```python
from build123d import *

# Parameters (mm, degrees)
SZKIC1_W                    = 32
SZKIC1_H                    = 25
DODANIE_WYCI_GNI_CIE1_DEPTH = 2
SZKIC2_W                    = 5.75
SZKIC2_H                    = 25
DODANIE_WYCI_GNI_CIE2_DEPTH = 3
SZKIC4_W                    = 11.75
SZKIC4_H                    = 5
SZKIC4_W_2                  = 6
SZKIC4_W_3                  = 5.75
DODANIE_WYCI_GNI_CIE3_DEPTH = 40
SZKIC5_R                    = 1.25
WYTNIJ_WYCI_GNI_CIE1_DEPTH  = 35
SZKIC7_R                    = 2
WYTNIJ_WYCI_GNI_CIE2_DEPTH  = 35
SFAZOWANIE1_SIZE            = 10
SFAZOWANIE2_SIZE            = 2


with BuildPart() as part:
    # Szkic1 → Dodanie-wyciągnięcie1 (new body)
    with BuildSketch(Plane.XY):
        Rectangle(SZKIC1_W, SZKIC1_H)
    extrude(amount=DODANIE_WYCI_GNI_CIE1_DEPTH)

    # Szkic2 → Dodanie-wyciągnięcie2 (add)
    with BuildSketch(Plane(origin=(0, 0, 0), x_dir=(-1, 0, 0), z_dir=(0, 0, -1))):
        with Locations((-13.125, 0)):
            Rectangle(SZKIC2_W, SZKIC2_H)
        with Locations((13.125, 0)):
            Rectangle(SZKIC2_W, SZKIC2_H)
    extrude(amount=DODANIE_WYCI_GNI_CIE2_DEPTH)

    # Szkic4 → Dodanie-wyciągnięcie3 (add)
    with BuildSketch(Plane(origin=(0, 0, -3), x_dir=(-1, 0, 0), z_dir=(0, 0, -1))):
        with Locations((-16.125, -10)):
            Rectangle(SZKIC4_W, SZKIC4_H)
        with Locations((19, -10)):
            Rectangle(SZKIC4_W_2, SZKIC4_H)
        with Locations((13.125, -10)):
            Rectangle(SZKIC4_W_3, SZKIC4_H)
    extrude(amount=-DODANIE_WYCI_GNI_CIE3_DEPTH)

    # Szkic5 → Wytnij-wyciągnięcie1 (cut)
    with BuildSketch(Plane.XY.offset(2)):
        with Locations((-13.5, 5.75)):
            Circle(SZKIC5_R)
        with Locations((-13.5, -2.25)):
            Circle(SZKIC5_R)
        with Locations((13.5, -2.25)):
            Circle(SZKIC5_R)
        with Locations((13.5, 5.75)):
            Circle(SZKIC5_R)
    extrude(amount=-WYTNIJ_WYCI_GNI_CIE1_DEPTH, mode=Mode.SUBTRACT)

    # Szkic7 → Wytnij-wyciągnięcie2 (cut)
    with BuildSketch(Plane(origin=(0, -7.5, 0), x_dir=(1, 0, 0), z_dir=(0, 1, 0))):
        with Locations(Location((18.5, -31.6, 0), (0, 0, 180))):
            Circle(SZKIC7_R)
        with Locations(Location((18.5, -18.6, 0), (0, 0, 180))):
            Circle(SZKIC7_R)
        with Locations(Location((-18.5, -25.6, 0), (0, 0, 180))):
            Circle(SZKIC7_R)
        with Locations(Location((-18.5, -12.6, 0), (0, 0, 180))):
            Circle(SZKIC7_R)
    extrude(amount=-WYTNIJ_WYCI_GNI_CIE2_DEPTH, mode=Mode.SUBTRACT)

    # Sfazowanie1
    # the kernel refuses this chamfer: 10 mm, written as the material it adds along each edge
    with BuildSketch(Plane(origin=(16, -7.5, -3), x_dir=(0.9996219169112968, -0.027495876610586317, 0), z_dir=(0, 0, 1))) as sfazowanie1_piece_1_section:
        Polygon((SFAZOWANIE1_SIZE * 0.999621916911, SFAZOWANIE1_SIZE * 0.0274958766106), (-SFAZOWANIE1_SIZE * 0.0274958766106, SFAZOWANIE1_SIZE * 0.999621916911), (0, 0), align=None)
    sfazowanie1_piece_1 = extrude(amount=5, mode=Mode.PRIVATE)
    sfazowanie1_piece_1 = split(sfazowanie1_piece_1, bisect_by=Plane(origin=(22, -3.749905405, -0.5), z_dir=(-1, 0, 0)), keep=Keep.TOP, mode=Mode.PRIVATE)
    add(sfazowanie1_piece_1)
    with BuildSketch(Plane(origin=(-16, -7.5, 2), x_dir=(-0.9996219169112968, -0.027495876610586403, 0), z_dir=(0, 0, -1))) as sfazowanie1_piece_2_section:
        Polygon((SFAZOWANIE1_SIZE * 0.999621916911, SFAZOWANIE1_SIZE * 0.0274958766106), (-SFAZOWANIE1_SIZE * 0.0274958766106, SFAZOWANIE1_SIZE * 0.999621916911), (0, 0), align=None)
    sfazowanie1_piece_2 = extrude(amount=5, mode=Mode.PRIVATE)
    sfazowanie1_piece_2 = split(sfazowanie1_piece_2, bisect_by=Plane(origin=(-22, -3.749905405, -0.5), z_dir=(1, 0, 0)), keep=Keep.TOP, mode=Mode.PRIVATE)
    add(sfazowanie1_piece_2)

    # Sfazowanie2
    sfazowanie2_edges = [part.edges().sort_by_distance(p)[0] for p in [
        (16.125, -7.5, 2),
        (-16.125, -7.5, 2),
    ]]
    chamfer(sfazowanie2_edges, length=SFAZOWANIE2_SIZE)


solid = part.part
```
Check sheet for the modelled part. Datum: model origin and axes. Units: mm. A direction names the side the tool comes from. Coordinates: 2 decimals unless noted, no trailing zeros. Order: outer loops, then holes, each group sorted by start corner. A loop starts at its lowest first (then second) coordinate and runs counter-clockwise, first axis right, second up. Notation, with made-up numbers: M -30,-34 L -22,-34 A13 cw -22,-29 Z; hole C 53,-8.5 d9. An arc over 180 degrees is marked long. One line per question, with ' | ' between items. Start each with the question number.
Item 1: Sectioned sample at B-B on x = 18.5. Record the cut outline in (y, z), and give its area (4 significant figures).
Item 2: Sectioned sample at C-C on z = 25.6. Record the cut outline in (x, y), and give its area (3 significant figures).
Item 3: Material ranges on line 1 (Z direction, x = 18.5, y = -11.2); line 2 (Y direction, x = 13.5, z = -1.05); line 3 (Z direction, x = -6.5, y = -6.75), recorded low to high.
Item 4: Sectioned sample at A-A on z = 5. Record the cut outline in (x, y).
Item 5: Mould release check, pull along X, two halves, no side actions. Record for faces 1 (the flat face through (-16, -10, 37)), 2 (the cylindrical face through (-13.77, 4.53, -0.46)), 3 (the flat face through (-19, -0.5, -0.5)): pulls with the +X half, pulls with the -X half, needs draft (parallel to the pull), parting line crosses it, or undercut.
Item 6: Gauge pin test, flat ends, axial feed: P1, Ø6.5, axis at x = -18.5, z = 25.6, coming from the -Y side; P2, Ø13, axis at x = -16, z = 16.5, coming from the +Y side; P3, Ø7.5, axis at x = -3, y = 3, coming from the +Z side; P4, Ø1.5, axis at y = 7, z = -1, coming from the +X side. Record the tip position at first contact, or that the pin passes through.
Item 7: Sectioned sample at D-D on y = 8. Record the cut outline in (x, z), and give its area (3 significant figures).
Item 8: Access from +Z, -Z, +X, -X, +Y, -Y to the whole of each face (thin tool, end or side, straight path). Record for faces 4 (the flat face through (-16, -7.5, 20)), 5 (the flat face through (0, 0, 2)), 6 (the flat face through (0, 0, 0)).
Answer below:
1) outline: M -12.5,-3 L 0,-3 L 0,2 L -5.5,2 L -7.5,4 L -7.5,16.6 L -12.5,16.6 Z; M -12.5,20.6 L -7.5,20.6 L -7.5,29.6 L -12.5,29.6 Z; M -12.5,33.6 L -7.5,33.6 L -7.5,37 L -12.5,37 Z | area: 199.5 mm^2
2) outline: M -22,-12.5 L -20.5,-12.5 L -20.5,-7.5 L -22,-7.5 Z; M -16.5,-12.5 L -10.25,-12.5 L -10.25,-7.5 L -16.5,-7.5 Z; M 10.25,-12.5 L 22,-12.5 L 22,-7.5 L 10.25,-7.5 Z | area: 97.5 mm^2
3) line 1: z = -3 to 16.6, 20.6 to 29.6, 33.6 to 37 | line 2: y = -12.5 to -3.5, -1 to 4.5, 7 to 12.5 | line 3: z = 0 to 2
4) outline: M -22,-12.5 L -10.25,-12.5 L -10.25,-7.5 L -22,-7.5 Z; M 10.25,-12.5 L 22,-12.5 L 22,-7.5 L 10.25,-7.5 Z
5) face 1: needs draft | face 2: undercut | face 3: pulls with the -X half
6) P1: stops at y = -12.5 | P2: stops at y = -7.5 | P3: stops at z = 2 | P4: stops at x = 16
7) outline: M -16,-3 L -10.25,-3 L -10.25,0 L 10.25,0 L 10.25,-3 L 16,-3 L 16,2 L -16,2 Z | area: 98.5 mm^2
8) face 4: +Z, +X, -X, +Y | face 5: +Z, +Y | face 6: -Z, +Y, -Y
